Could you check a few things on this model? Use its own coordinates, in mm. Give positions to 0.01 mm unless a question says otherwise; leave off trailing zeros. Loops run counter-clockwise (first coordinate to the right, second up) from the corner with the lowest first, then second, coordinate; pieces in that order, holes last. Notation, with made-up numbers: (-32.75, -7) - (-11.75, -7) arc R32 ccw to (-11.75, 32) - close; hole circle Ø6 at (-6.75, 5.5). An arc over 180 degrees is marked (long way). Use CSV: the item, a comma, the result in double quotes.
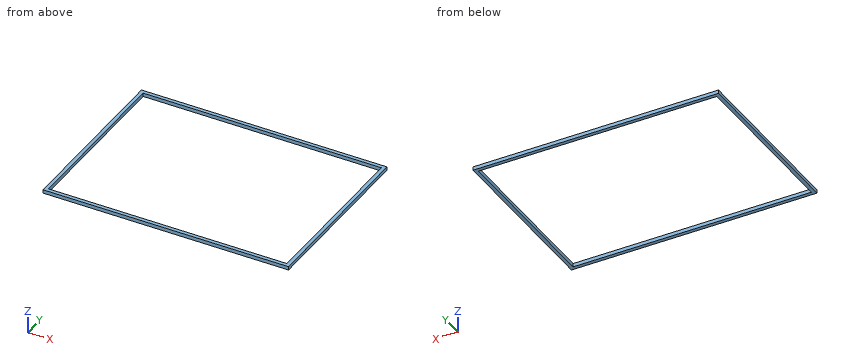
from build123d import *

# Parameters (mm, degrees)
F0_W     = 25.9512081146
F0_H     = 25.8589489582
F0_W_2   = 292.5098538399
F0_H_2   = 1230.8580875397
F0_W_3   = 26.0652303696
F0_H_3   = 25.9829635022
F0_W_4   = 26.0652527213
F0_W_5   = 779.060781002
F1_DEPTH = 25.4


with BuildPart() as f1:
    # F0 (on Top) → F1 (new body)
    with BuildSketch(Plane.XY):
        with Locations((-834.7059197426, 157.3672643961)):
            Rectangle(F0_W, F0_H)
        with Locations((-675.4753887653, 157.3672643961)):
            Rectangle(F0_W_2, F0_H)
        with Locations((-834.7059197426, -470.9912538528)):
            Rectangle(F0_W, F0_H_2)
        with Locations((-516.1878466606, 157.3672643961)):
            Rectangle(F0_W_3, F0_H)
        with Locations((-834.7059197426, -1099.4117793738)):
            Rectangle(F0_W, F0_H_3)
        Polygon((99.2412343621, 170.2967388751), (-503.1552314758, 170.2967388751), (-503.1552314758, 144.437789917), (-225.1261025667, 144.437789917), (-199.060857296, 144.437789917), (99.2412343621, 144.437789917), align=None)
        with Locations((-675.4753887653, -1099.4117793738)):
            Rectangle(F0_W_2, F0_H_3)
        with Locations((112.2738607228, 157.3672643961)):
            Rectangle(F0_W_4, F0_H)
        with Locations((-516.1878466606, -1099.4117793738)):
            Rectangle(F0_W_3, F0_H_3)
        with Locations((514.8368775845, 157.3672643961)):
            Rectangle(F0_W_5, F0_H)
        Polygon((-225.1261025667, -1086.4202976227), (-503.1552314758, -1086.4202976227), (-503.1552314758, -1112.4032611249), (99.2412343621, -1112.4032611249), (99.2412343621, -1086.4202976227), (-199.060857296, -1086.4202976227), align=None)
        with Locations((917.3428721428, 157.3672643961)):
            Rectangle(F0_W, F0_H)
        with Locations((112.2738607228, -1099.4117793738)):
            Rectangle(F0_W_4, F0_H_3)
        with Locations((917.3428721428, -470.9912538528)):
            Rectangle(F0_W, F0_H_2)
        with Locations((514.8368775845, -1099.4117793738)):
            Rectangle(F0_W_5, F0_H_3)
        with Locations((917.3428721428, -1099.4117793738)):
            Rectangle(F0_W, F0_H_3)
    extrude(amount=F1_DEPTH)


solid = f1.part
1) Suppose I cut it at B-B (x = -696). Please give me the cut outline in (y, z), plus the area to 3 significant figures.
Answer below:
outline,"(-1112.4, 0) - (-1086.42, 0) - (-1086.42, 25.4) - (-1112.4, 25.4) - close; (144.44, 0) - (170.3, 0) - (170.3, 25.4) - (144.44, 25.4) - close"
area,"1,320 mm2"
2) I need wall thicknesses on line 1 along X through (y, z) = (-849, 22); line 2 along Y through (x, z) = (-551, 11.25). Which ranges of each line are inside material? Lowest first, please.
Answer below:
line 1,"x = -847.68 to -821.73, 904.37 to 930.32"
line 2,"y = -1112.4 to -1086.42, 144.44 to 170.3"
3) Suppose I cut it at A-A (y = -349). Please give me the cut outline in (x, z), plus the area to 3 significant figures.
Answer below:
outline,"(-847.68, 0) - (-821.73, 0) - (-821.73, 25.4) - (-847.68, 25.4) - close; (904.37, 0) - (930.32, 0) - (930.32, 25.4) - (904.37, 25.4) - close"
area,"1,320 mm2"
4) Suppose I cut it at C-C (z = 4.25). Please give me the cut outline in (x, y).
Answer below:
outline,"(-847.68, -1112.4) - (930.32, -1112.4) - (930.32, 170.3) - (-847.68, 170.3) - close; hole (-821.73, -1086.42) - (904.37, -1086.42) - (904.37, 144.44) - (-821.73, 144.44) - close"
